Build history of the part. All positions in model axes, mm. A direction names the side the tool comes from. Round coordinates to 2 decimals unless told otherwise and drop trailing zeros. Order: outer loops, then holes, each group sorted by start corner. A loop starts at its lowest first (then second) coordinate and runs counter-clockwise, first axis right, second up. Notation, with made-up numbers: M 59.25,58.25 L 96.25,58.25 A5 cw 96.25,65.25 Z; hole C 84.25,14.25 d6. An arc over 180 degrees is marked long. Use CSV: the item, a comma, the result in double quotes.
from build123d import *

# Parameters (mm, degrees)
SKETCH3_R           = 1.5
SKETCH3_R_2         = 1.25
BOSS_EXTRUDE1_DEPTH = 4
BOSS_EXTRUDE2_DEPTH = 40
BOSS_EXTRUDE5_DEPTH = 50
BOSS_EXTRUDE6_REACH = 91.057
CUT_EXTRUDE2_DEPTH  = 90.057130972
BOSS_EXTRUDE7_DEPTH = 2.3094


with BuildPart() as part:
    # Sketch3 → Boss-Extrude1 (new body)
    with BuildSketch(Plane.XY):
        with BuildLine():
            Line((-53.55, 25), (-53.55, -25))
            ThreePointArc((-53.55, -25), (-52.085533906, -28.535533906), (-48.55, -30))
            Line((-48.55, -30), (49.15, -30))
            ThreePointArc((49.15, -30), (52.685533906, -28.535533906), (54.15, -25))
            Line((54.15, -25), (54.15, 25))
            ThreePointArc((54.15, 25), (52.685533906, 28.535533906), (49.15, 30))
            Line((49.15, 30), (-48.55, 30))
            ThreePointArc((-48.55, 30), (-52.085533906, 28.535533906), (-53.55, 25))
        make_face()
        with Locations((-39.7, 27.5)):
            Circle(SKETCH3_R, mode=Mode.SUBTRACT)
        with Locations((40.3, 27.5)):
            Circle(SKETCH3_R, mode=Mode.SUBTRACT)
        with Locations((40.3, -27.5)):
            Circle(SKETCH3_R, mode=Mode.SUBTRACT)
        with Locations((0.3, -27.5)):
            Circle(SKETCH3_R, mode=Mode.SUBTRACT)
        with Locations((-50.65, -12)):
            Circle(SKETCH3_R, mode=Mode.SUBTRACT)
        with Locations((-50.65, 12)):
            Circle(SKETCH3_R, mode=Mode.SUBTRACT)
        with Locations((-39.7, -27.5)):
            Circle(SKETCH3_R, mode=Mode.SUBTRACT)
        with Locations((0.3, 27.5)):
            Circle(SKETCH3_R, mode=Mode.SUBTRACT)
        with Locations((50.65, 0)):
            Circle(SKETCH3_R_2, mode=Mode.SUBTRACT)
        with BuildLine():
            Line((-48.15, 22), (-48.15, -22))
            ThreePointArc((-48.15, -22), (-47.271320344, -24.121320344), (-45.15, -25))
            Line((-45.15, -25), (45.15, -25))
            ThreePointArc((45.15, -25), (46.564213562, -24.414213562), (47.15, -23))
            Line((47.15, -23), (47.15, 23))
            ThreePointArc((47.15, 23), (46.564213562, 24.414213562), (45.15, 25))
            Line((45.15, 25), (-45.15, 25))
            ThreePointArc((-45.15, 25), (-47.271320344, 24.121320344), (-48.15, 22))
        make_face(mode=Mode.SUBTRACT)
    extrude(amount=BOSS_EXTRUDE1_DEPTH)

    # Sketch5 → Boss-Extrude2 (add)
    # profile 1 of 3: a face of its own
    with BuildSketch(Plane.XY.offset(4)):
        Polygon((-17.693593539, 30), (-13.074791386, 38), (-17.693593539, 46), (-26.931197846, 46), (-31.55, 38), (-26.931197846, 30), align=None)
        Polygon((-18.848294078, 44), (-15.384192463, 38), (-18.848294078, 32), (-25.776497308, 32), (-29.240598923, 38), (-25.776497308, 44), align=None, mode=Mode.SUBTRACT)
    # profile 2 of 3: a face of its own
    with BuildSketch(Plane.XY.offset(4)):
        Polygon((-13.074791386, 30), (-13.074791386, 38), (-17.693593539, 30), align=None)
    # profile 3 of 3: a face of its own
    with BuildSketch(Plane.XY.offset(4)):
        Polygon((-31.55, 30), (-26.931197846, 30), (-31.55, 38), align=None)
    extrude(amount=-BOSS_EXTRUDE2_DEPTH)

    # Sketch8 → Boss-Extrude5 (add)
    with BuildSketch(Plane(origin=(-13.074791386, 0, 0), x_dir=(0, 0, -1), z_dir=(1, 0, 0))):
        Polygon((0, 30), (0.618802154, 30), (-4, 38), (-4, 30), align=None)
        Polygon((9.856406461, 30), (14.475208614, 38), (12.165807537, 38), (8.701705922, 32), (1.773502692, 32), (-1.690598923, 38), (-4, 38), (0.618802154, 30), align=None)
        Polygon((14.475208614, 30), (14.475208614, 38), (9.856406461, 30), align=None)
        Polygon((12.165807537, 38), (14.475208614, 38), (9.856406461, 46), (0.618802154, 46), (-4, 38), (-1.690598923, 38), (1.773502692, 44), (8.701705922, 44), align=None)
    extrude(amount=BOSS_EXTRUDE5_DEPTH)

    # Boss-Extrude6: up to this face of the body (flat: up to its plane)
    boss_extrude6_end = Plane(part.part.faces().sort_by_distance((-15.384192463, 42, -16))[0])
    # Sketch8<3> → Boss-Extrude6 (add, up to the picked face)
    with BuildSketch(Plane(origin=(-13.074791386, 0, 0), x_dir=(0, 0, -1), z_dir=(1, 0, 0)), mode=Mode.PRIVATE) as boss_extrude6_sk1:
        Polygon((12.165807537, 38), (14.475208614, 38), (9.856406461, 46), (0.618802154, 46), (-4, 38), (-1.690598923, 38), (1.773502692, 44), (8.701705922, 44), align=None)
    boss_extrude6_tool1 = split(extrude(boss_extrude6_sk1.sketch, amount=-BOSS_EXTRUDE6_REACH, mode=Mode.PRIVATE), bisect_by=boss_extrude6_end, keep=Keep.BOTH, mode=Mode.PRIVATE)
    add(boss_extrude6_tool1.solids().sort_by(Axis((-13.074791, 38.201329, -13.320508), (-1, 0, 0)))[0])

    # Sketch8<4> → Cut-Extrude2 (cut, through all)
    with BuildSketch(Plane(origin=(-13.074791386, 0, 0), x_dir=(0, 0, -1), z_dir=(1, 0, 0))):
        Polygon((-1.690598923, 38), (12.165807537, 38), (8.701705922, 44), (1.773502692, 44), align=None)
        Polygon((8.701705922, 32), (12.165807537, 38), (-1.690598923, 38), (1.773502692, 32), align=None)
    extrude(amount=-CUT_EXTRUDE2_DEPTH, mode=Mode.SUBTRACT)

    # Sketch5<3> → Boss-Extrude7 (add)
    with BuildSketch(Plane.XY.offset(4)):
        Polygon((-25.776497308, 32), (-18.848294078, 32), (-15.384192463, 38), (-18.848294078, 44), (-25.776497308, 44), (-29.240598923, 38), align=None)
    extrude(amount=-BOSS_EXTRUDE7_DEPTH)


solid = part.part
(1) Wall check: line 1 (Y direction, x = -39.7, z = 3.1); line 2 (X direction, y = -27, z = 2); line 3 (Y direction, x = -50.65, z = 1.2). Give the ranges that are in metal, low to high. Write a range as from..to.
Answer block:
line 1,"y = -30..-29, -26..-25, 25..26, 29..30"
line 2,"x = -53.13..-41.11, -38.29..-1.11, 1.71..38.89, 41.71..53.73"
line 3,"y = -29.54..-13.5, -10.5..10.5, 13.5..29.54"
(2) Cut at C-C, the plane x = 16. Give the cut face in (y, z).
Answer block:
outline,"M -30,0 L -25,0 L -25,4 L -30,4 Z; M 25,0 L 30,0 L 30,-14.48 L 38,-14.48 L 46,-9.86 L 46,-0.62 L 38,4 L 25,4 Z; hole M 32,-8.7 L 38,-12.17 L 44,-8.7 L 44,-1.77 L 38,1.69 L 32,-1.77 Z"
(3) Cut at A-A, the plane x = 0.3. Give the cut face in (y, z), and give its area (3 significant figures).
Answer block:
outline,"M -30,0 L -29,0 L -29,4 L -30,4 Z; M -26,0 L -25,0 L -25,4 L -26,4 Z; M 25,0 L 26,0 L 26,4 L 25,4 Z; M 29,0 L 30,0 L 30,-14.48 L 38,-14.48 L 46,-9.86 L 46,-0.62 L 38,4 L 29,4 Z; hole M 32,-8.7 L 38,-12.17 L 44,-8.7 L 44,-1.77 L 38,1.69 L 32,-1.77 Z"
area,"150 mm²"
(4) Tool access for faces 4 (the face through (8.648, 35.042, -10.458)), 5 (the face through (-17.092, 35.042, -22.16)), 6 (the face through (-47.25, 24.14, 1.97)), 7 (the face through (-0.5, 25.4, 4)): list every direction of +Z, -Z, +X, -X, +Y, -Y with a clear straight run to the whole face (end or side of a thin tool).
Answer block:
face 4,"+X, -X"
face 5,"-Z"
face 6,"+Z, -Z"
face 7,"+Z, +X, -X, +Y, -Y"
(5) Cut at B-B, the plane y = 0. Give the cut face in (x, z).
Answer block:
outline,"M -53.55,0 L -48.15,0 L -48.15,4 L -53.55,4 Z; M 47.15,0 L 49.4,0 L 49.4,4 L 47.15,4 Z; M 51.9,0 L 54.15,0 L 54.15,4 L 51.9,4 Z"
(6) Drop flat-ended pins along their axis: pin 1 (18 mm diameter, centred on x = 15.5, z = -22.5, fed in from -Y); pin 2 (1.8 mm diameter, centred on x = 0.3, y = -27.5, fed in from -Z); pin 3 (3 mm diameter, centred on x = -13, z = 3, fed in from +Y); pin 4 (4 mm diameter, centred on y = 35.5, z = -11.5, fed in from -X). Give the stop position or say it passes through.
Answer block:
pin 1,"stops at y = 30"
pin 2,"passes through"
pin 3,"stops at y = 42.33"
pin 4,"stops at x = -31.55"
(7) Two-plate mould, pull along Z, no slides. Class faces 1 (the face through (-5, 44, -7)), 2 (the face through (9.998, 42.056, 1.658)), 3 (the face through (1, 25, 2)): released by +Z, released by -Z, zero draft, split by the parting line, or undercut.
Answer block:
face 1,"undercut"
face 2,"released by +Z"
face 3,"zero draft"
(8) Cut at D-D, the plane z = -24.5. Give the cut face in (x, y).
Answer block:
outline,"M -31.55,30 L -13.07,30 L -13.07,38 L -17.69,46 L -26.93,46 L -31.55,38 Z; hole M -29.24,38 L -25.78,32 L -18.85,32 L -15.38,38 L -18.85,44 L -25.78,44 Z"
